Verification items for the finished model (mm, model axes). A direction names the side the tool comes from. Round coordinates to 2 decimals unless told otherwise and drop trailing zeros. Write each loop counter-clockwise with the first axis right and the second up, starting at its lowest first coordinate (ties: lowest second). Pieces come first, ordered by that corner, then holes. Notation, with made-up numbers: (73, 80.25) -> (122, 80.25) arc R21 cw to (122, 100.25) -> close; hole circle Ø6 at (-9.75, -26.5). An arc over 180 degrees is marked (long way). Answer as a JSON object with one key per item and string values. Group by question number.
(1) Set-up check for faces 1 (the face through (41.784, 0.783, 3.999)), 2 (the face through (56.2, 0.78, -18.14)): record each of +Z, -Z, +X, -X, +Y, -Y from which the full face is reachable in a straight line by a thin tool's end or side.
(2) Draft check along Z on faces 3 (the face through (5.31, 0.78, -5.44)), 4 (the face through (39.91, 0.78, 13.03)), 5 (the face through (20, 1, 19.05)), 6 (the face through (57.15, 1, -8)). Enter one of: released by +Z, released by -Z, zero draft, split by the parting line, or undercut.
(3) Gauge pin test, flat ends, axial feed: pin 1 Ø10 at (x, z) = (34, -2) entering from +Y; pin 2 Ø0.8 at (x, y) = (26, 1) entering from -Z (3 decimals). Record the tip position at first contact, or that the pin passes through.
(4) Sectioned sample at B-B on x = 0. Record the cut outline in (y, z), and give its area (3 significant figures).
(5) Scan lines: L1, parallel to Z at x = 0, y = 0.5; L2, parallel to Z at x = 50.8, y = 0.5; L3, parallel to X at y = 1.25, z = -1.5. Record each from-to range of solid material in increasing order. Write a range as from..to.
(6) Sectioned sample at A-A on z = -12.7. Record the cut outline in (x, y).
(7) Sectioned sample at C-C on y = 0.45. Count the separate pieces of the cut face and the enclosed holes in it, and give its area (3 significant figures).
Autodesk Inventor part; units mm, degrees
ref_plane "YZ Plane" through (0, 0, 0) normal (1, 0, 0) x (0, 1, 0)
ref_plane "XZ Plane" through (0, 0, 0) normal (0, 1, 0) x (-1, 0, 0)
ref_plane "XY Plane" through (0, 0, 0) normal (0, 0, 1) x (1, 0, 0)
sketch "main" plane through (0, 0, 0) normal (0, 0, 1) x (1, 0, 0)
  point P0 (-4.8343, 8.0815)
sketch "Sketch1" plane through (0, 0, 0) normal (0, 1, 0) x (-1, 0, 0)
  circle A0 centre (0, 0) radius 2.0955
  circle A1 centre (0, 12.7) radius 2.0955
  circle A2 centre (-50.8, 0) radius 2.0955
  line L0 (6.4379, -3.175) -> (6.4379, 15.875)
  line L1 (3.2629, 19.05) -> (-6.2621, 19.05)
  line L2 (-6.2621, 6.35) -> (-6.2621, -3.175)
  line L3 (-3.0871, -6.35) -> (3.2629, -6.35)
  line L4 (3.2629, 19.05) -> (-44.0264, 19.05)
  line L5 (-44.45, -15.875) -> (-44.45, 0)
  line L6 (-9.4371, 9.525) -> (-36.4008, 9.525)
  line L7 (-57.15, 0) -> (-57.15, -15.875)
  line L8 (-53.975, -19.05) -> (-47.625, -19.05)
  arc A3 (3.2629, -6.35) -> (6.4379, -3.175) centre (3.2629, -3.175) ccw
  arc A4 (-6.2621, -3.175) -> (-3.0871, -6.35) centre (-3.0871, -3.175) ccw
  arc A5 (6.4379, 15.875) -> (3.2629, 19.05) centre (3.2629, 15.875) ccw
  arc A6 (-47.625, -19.05) -> (-44.45, -15.875) centre (-47.625, -15.875) ccw
  arc A7 (-57.15, -15.875) -> (-53.975, -19.05) centre (-53.975, -15.875) ccw
  arc A8 (-6.2621, 6.35) -> (-9.4371, 9.525) centre (-9.4371, 6.35) ccw
  circle A9 centre (-41.0406, 14.7955) radius 2.0955
  circle A10 centre (-50.8, -12.7) radius 2.0955
  line L9 (-44.45, 0) -> (-39.0426, 8.1112)
  arc A11 (-55.9385, 3.7307) -> (-57.15, 0) centre (-50.8, 0) ccw
  line L10 (-56.2201, 3.3084) -> (-46.6682, 17.6362)
  arc A12 (-44.0264, 19.05) -> (-46.6682, 17.6362) centre (-44.0264, 15.875) ccw
  arc A13 (-36.4008, 9.525) -> (-39.0426, 8.1112) centre (-36.4008, 6.35) ccw
  point P0 (-44.45, -19.05)
  point P1 (-57.15, -19.05)
  point P2 (-50.8, -19.05)
  dimension "d17" = 4.191
  dimension "d19" = 12.7
  dimension "d20" = 3.175
  dimension "d21" = 3.175
  dimension "d22" = 4.191
  dimension "d23" = 6.35
  dimension "d24" = 3.175
extrude "Extrusion1" add sketch "Sketch1" along normal blind 1.5875
equation "\"BendRadius\" = Thickness"
equation "\"BendReliefWidth\" = Thickness"
equation "\"BendReliefDepth\" = 0.5 * Thickness"
equation "\"CornerReliefSize\" = 4 * Thickness"
equation "\"MinimumRemnant\" = 2 * Thickness"
equation "\"TransitionRadius\" = BendRadius"
equation "\"JacobiRadiusSize\" = BendRadius"
equation "\"GapSize\" = Thickness"
properties part number "MOGO Funnel" material "Acetal Resin, White"
Computed values:
{
 "1": {"face 1": "-Z, +Y, -Y", "face 2": "-Z, +X, +Y, -Y"},
 "2": {"face 3": "released by -Z", "face 4": "undercut", "face 5": "released by +Z", "face 6": "zero draft"},
 "3": {"pin 1": "through", "pin 2": "z = 9.525"},
 "4": {"outline": "(0, -6.35) -> (1.59, -6.35) -> (1.59, -2.1) -> (0, -2.1) -> close; (0, 2.1) -> (1.59, 2.1) -> (1.59, 10.6) -> (0, 10.6) -> close; (0, 14.8) -> (1.59, 14.8) -> (1.59, 19.05) -> (0, 19.05) -> close", "area": "27.0 mm2"},
 "5": {"L1": "-6.35..-2.1, 2.1..10.6, 14.8..19.05", "L2": "-19.05..-14.8, -10.6..-2.1, 2.1..11.44", "L3": "-6.44..-1.46, 1.46..6.26, 44.45..49.34, 52.26..57.15"},
 "6": {"outline": "(44.45, 0) -> (48.7, 0) -> (48.7, 1.59) -> (44.45, 1.59) -> close; (52.9, 0) -> (57.15, 0) -> (57.15, 1.59) -> (52.9, 1.59) -> close"},
 "7": {"separate pieces": "1", "enclosed holes": "5", "area": "1,020 mm2"}
}
